from build123d import *

# Parameters (mm, degrees)
SKETCH_2_W          = 106
SKETCH_2_H          = 100
EXTRUDE_1_DEPTH     = 10
SKETCH_3_R          = 2
EXTRUDE_2_DEPTH     = 10
EXTRUDE_3_DEPTH     = 17
SKETCH_5_W          = 68
SKETCH_5_H          = 40
CUT_EXTRUDE_1_DEPTH = 20
SKETCH_6_W          = 46
SKETCH_6_H          = 32
CUT_EXTRUDE_2_DEPTH = 20
FILLET_1_R          = 3
FILLET_2_R          = 5


with BuildPart() as part:
    # 草图2 → 凸台-拉伸1 (new body)
    with BuildSketch(Plane(origin=(0, 0, 0), x_dir=(1, 0, 0), z_dir=(0, 1, 0))):
        Rectangle(SKETCH_2_W, SKETCH_2_H)
    extrude(amount=EXTRUDE_1_DEPTH)

    # 草图3 → 凸台-拉伸2 (add)
    with BuildSketch(Plane.XZ):
        with Locations(Location((-32, 43, 0), (0, 0, 270))):
            Circle(SKETCH_3_R)
        with Locations(Location((32, 43, 0), (0, 0, 270))):
            Circle(SKETCH_3_R)
    extrude(amount=EXTRUDE_2_DEPTH)

    # 草图4 → 凸台-拉伸3 (add)
    with BuildSketch(Plane.XZ):
        Polygon((-53, 50), (-43, 50), (-43, 34), (43, 34), (43, 50), (53, 50), (53, -50), (43, -50), (-43, -50), (-53, -50), align=None)
    extrude(amount=EXTRUDE_3_DEPTH)

    # 草图5 → 切除-拉伸1 (cut)
    with BuildSketch(Plane(origin=(0, 10, 0), x_dir=(1, 0, 0), z_dir=(0, 1, 0))):
        with Locations((0, 25)):
            Rectangle(SKETCH_5_W, SKETCH_5_H)
    extrude(amount=-CUT_EXTRUDE_1_DEPTH, mode=Mode.SUBTRACT)

    # 草图6 → 切除-拉伸2 (cut)
    with BuildSketch(Plane.XZ):
        with Locations((0, 50)):
            Rectangle(SKETCH_6_W, SKETCH_6_H)
    extrude(amount=-CUT_EXTRUDE_2_DEPTH, mode=Mode.SUBTRACT)

    # 圆角1
    fillet_1_edges = [part.edges().sort_by_distance(p)[0] for p in [
        (-32, 0, 45),
        (32, 0, 45),
    ]]
    fillet(fillet_1_edges, radius=FILLET_1_R)

    # 圆角2
    fillet_2_edges = [part.edges().sort_by_distance(p)[0] for p in [
        (-53, 10, 0),
        (-38, 10, 50),
        (53, 10, 0),
        (38, 10, 50),
        (53, -3.5, 50),
        (-53, -3.5, 50),
        (-53, -3.5, -50),
        (53, -3.5, -50),
        (0, 10, -50),
    ]]
    fillet(fillet_2_edges, radius=FILLET_2_R - 0.0001)  # a hair under: the kernel refuses the full size


solid = part.part
Design review of the part built by this model. Coordinates are the model's own, in mm. A direction names the side the tool comes from. Coordinates: 2 decimals unless noted, no trailing zeros. Write each loop counter-clockwise with the first axis right and the second up, starting at its lowest first coordinate (ties: lowest second). Pieces come first, ordered by that corner, then holes. Notation, with made-up numbers: (56, 71) - (77, 71) arc R23 ccw to (77, 95) - close; hole circle Ø11 at (85.25, -34.75). An arc over 180 degrees is marked (long way). Use one line per item in the form item = value.
Q1. Consider section C-C (y = 2.5). Write out the cut boundary in (x, z), plus the area to 3 significant figures.
Taken from the geometry:
outline = (-53, -45) arc R5 ccw to (-48, -50) - (48, -50) arc R5 ccw to (53, -45) - (53, 45) arc R5 ccw to (48, 50) - (23, 50) - (23, 34) - (-23, 34) - (-23, 50) - (-48, 50) arc R5 ccw to (-53, 45) - close; hole (-34, -45) - (34, -45) - (34, -5) - (-34, -5) - close
area = 7,120 mm^2
Q2. Consider section B-B (z = 43). Write out the cut boundary in (x, y).
Taken from the geometry:
outline = (-53, -17) - (-43, -17) - (-43, 0) - (-37, 0) arc R3 cw to (-34, -3) - (-34, -10) - (-30, -10) - (-30, -3) arc R3 cw to (-27, 0) - (-23, 0) - (-23, 10) - (-48, 10) arc R5 ccw to (-53, 5) - close; (23, 0) - (27, 0) arc R3 cw to (30, -3) - (30, -10) - (34, -10) - (34, -3) arc R3 cw to (37, 0) - (43, 0) - (43, -17) - (53, -17) - (53, 5) arc R5 ccw to (48, 10) - (23, 10) - close
Q3. Machinability: for faces 1 (the flat face through (0, 0, -45)), 2 (the flat face through (-43, -8, 42)), 3 (the flat face through (-23, 5, 42)), 4 (the flat face through (-35, 0, 38)), which of the approach directions +Z, -Z, +X, -X, +Y, -Y give a long, thin tool a straight path to every point of the face, cutting with its end or side? Answer none if there is none.
Taken from the geometry:
face_1 = +Y
face_2 = +Z, -Y
face_3 = +Z, +Y, -Y
face_4 = -Y
Q4. For probe 1 along Z at (x, y) = (20, -7.75); probe 2 along X at (y, z) = (-7, -9); probe 3 along X at (y, z) = (-5.25, 41.5), list the stretches that pass through material, from the lowest coordinate up.
Taken from the geometry:
probe_1 = -50 to -45, -5 to 34
probe_2 = -53 to -34, 34 to 53
probe_3 = -53 to -43, -33.32 to -30.68, 30.68 to 33.32, 43 to 53
Q5. Insertion check: pin 1 Ø5 at (x, y) = (3.5, -12) entering from +Z; pin 2 Ø8 at (x, z) = (34, 45.5) entering from -Y; pin 3 Ø2 at (x, y) = (-36.5, -0.5) entering from +Z; pin 4 Ø1 at (y, z) = (6.5, 16) entering from +X. Each pin has a flat end and moves straight along its axis. Give the tip position at first contact, or say it passes through.
Taken from the geometry:
pin_1 = 34
pin_2 = -10
pin_3 = 50
pin_4 = 52.9
Q6. The part is to be moulded in two halves that separate along X. For faces 5 (the flat face through (41, 1, 50)), 6 (the cylindrical face through (51, 9, -1)), 7 (the cylindrical face through (-52, -6, -48)), 8 (the flat face through (35, 0, 38)), say which applies: +X half, -X half, draft (parallel to the pull), parting line (faces both ways), or undercut.
Taken from the geometry:
face_5 = draft
face_6 = +X half
face_7 = -X half
face_8 = undercut
Q7. Consider section A-A (y = -6.25). Write out the cut boundary in (x, z), plus the area to 3 significant figures.
Taken from the geometry:
outline = (-53, -45) arc R5 ccw to (-48, -50) - (48, -50) arc R5 ccw to (53, -45) - (53, 45) arc R5 ccw to (48, 50) - (43, 50) - (43, 34) - (-43, 34) - (-43, 50) - (-48, 50) arc R5 ccw to (-53, 45) - close; circle Ø4 at (-32, 43); circle Ø4 at (32, 43); hole (-34, -45) - (34, -45) - (34, -5) - (-34, -5) - close
area = 6,510 mm^2
